Geometry check sheet. Reference: the model listing, model coordinates, mm. A direction names the side the tool comes from. Give positions to 0.01 mm unless a question says otherwise; leave off trailing zeros. Write each loop counter-clockwise with the first axis right and the second up, starting at its lowest first coordinate (ties: lowest second). Pieces come first, ordered by that corner, then holes. Notation, with made-up numbers: (71.5, 35) -> (119.5, 35) arc R20 cw to (119.5, 60) -> close; hole circle Ø11 at (60.25, -7). An arc over 180 degrees is marked (long way). One line per item, written item: value.
from build123d import *

# Parameters (mm, degrees)
CROQUIS1_R              = 2
SALIENTE_EXTRUIR1_DEPTH = 2.5
REDONDEO6_R             = 3
REDONDEO7_R             = 3
REDONDEO8_R             = 3


with BuildPart() as part:
    # Croquis1 → Saliente-Extruir1 (new body)
    with BuildSketch(Plane.XY):
        with BuildLine():
            Line((-15, 20.15), (-17.5, 20.15))
            Line((-17.5, 20.15), (-17.5, 15.15))
            Line((-17.5, 15.15), (-15, 15.15))
            Line((-15, 15.15), (-15, 10.15))
            Line((-15, 10.15), (-17.5, 10.15))
            Line((-17.5, 10.15), (-17.5, 0.15))
            Line((-17.5, 0.15), (-15, 0.15))
            Line((-15, 0.15), (-15, -9.85))
            Line((-15, -9.85), (-17.5, -9.85))
            Line((-17.5, -9.85), (-17.5, -19.85))
            Line((-17.5, -19.85), (-15, -19.85))
            Line((-15, -19.85), (-15, -24.85))
            Line((-15, -24.85), (-17.5, -24.85))
            Line((-17.5, -24.85), (-17.5, -29.85))
            Line((-17.5, -29.85), (-15, -29.85))
            Line((-15, -29.85), (15, -29.85))
            Line((15, -29.85), (17.5, -29.85))
            Line((17.5, -29.85), (17.5, -24.85))
            Line((17.5, -24.85), (15, -24.85))
            Line((15, -24.85), (15, -19.85))
            Line((15, -19.85), (17.5, -19.85))
            Line((17.5, -19.85), (17.5, -9.85))
            Line((17.5, -9.85), (15, -9.85))
            Line((15, -9.85), (15, 0.15))
            Line((15, 0.15), (17.5, 0.15))
            Line((17.5, 0.15), (17.5, 10.15))
            Line((17.5, 10.15), (15, 10.15))
            Line((15, 10.15), (15, 15.15))
            Line((15, 15.15), (17.5, 15.15))
            Line((17.5, 15.15), (17.5, 20.15))
            Line((17.5, 20.15), (15, 20.15))
            ThreePointArc((15, 20.15), (0, 35.15), (-15, 20.15))
        make_face()
        with Locations((-5, 24.315)):
            Circle(CROQUIS1_R, mode=Mode.SUBTRACT)
        with Locations((5, 24.315)):
            Circle(CROQUIS1_R, mode=Mode.SUBTRACT)
        with Locations((-5, -24.315)):
            Circle(CROQUIS1_R, mode=Mode.SUBTRACT)
        with Locations((5, -24.315)):
            Circle(CROQUIS1_R, mode=Mode.SUBTRACT)
        Polygon((-9.75, 20.15), (-1.5, 20.15), (-1.5, 26.15), (1.5, 26.15), (1.5, 20.15), (9.75, 20.15), (9.75, -20.15), (1.5, -20.15), (1.5, -26.15), (-1.5, -26.15), (-1.5, -20.15), (-9.75, -20.15), align=None, mode=Mode.SUBTRACT)
    extrude(amount=SALIENTE_EXTRUIR1_DEPTH)

    # Redondeo6
    redondeo6_edges = [part.edges().sort_by_distance(p)[0] for p in [
        (-1.5, -20.15, 1.25),
    ]]
    fillet(redondeo6_edges, radius=REDONDEO6_R)

    # Redondeo7
    redondeo7_edges = [part.edges().sort_by_distance(p)[0] for p in [
        (1.5, -20.15, 1.25),
    ]]
    fillet(redondeo7_edges, radius=REDONDEO7_R)

    # Redondeo8
    redondeo8_edges = [part.edges().sort_by_distance(p)[0] for p in [
        (1.5, 20.15, 1.25),
        (-1.5, 20.15, 1.25),
    ]]
    fillet(redondeo8_edges, radius=REDONDEO8_R)


solid = part.part
1) Sectioned sample at C-C on z = 0.4. Give the number of separate pieces and of enclosed holes in the cut face, plus the area to 3 significant figures.
Verdict:
separate pieces: 1
enclosed holes: 5
area: 1,120 mm^2
2) Tool access check on faces 1 (the flat face through (-16, 0.15, 1)), 2 (the flat face through (15, -5, 1)), 3 (the flat face through (-12, 3, 2.5)), 4 (the flat face through (0, -26.15, 1)). Record the directions out of +Z, -Z, +X, -X, +Y, -Y that give a thin tool (end or side, any length) a straight path to the whole face; none if there is none.
Verdict:
face 1: +Z, -Z, -X
face 2: +Z, -Z, +X
face 3: +Z, +X, -X, +Y, -Y
face 4: +Z, -Z
3) Sectioned sample at A-A on x = 0. Record the cut outline in (y, z), plus the area to 4 significant figures.
Verdict:
outline: (-29.85, 0) -> (-26.15, 0) -> (-26.15, 2.5) -> (-29.85, 2.5) -> close; (26.15, 0) -> (35.15, 0) -> (35.15, 2.5) -> (26.15, 2.5) -> close
area: 31.75 mm^2
4) Scan lines: probe 1 along Y at (x, z) = (15.5, 1); probe 2 along X at (y, z) = (-2.5, 0.25); probe 3 along X at (y, z) = (24.5, 1.9). Record each from-to range of solid material in increasing order.
Verdict:
probe 1: -29.85 to -24.85, -19.85 to -9.85, 0.15 to 10.15, 15.15 to 20.15
probe 2: -15 to -9.75, 9.75 to 15
probe 3: -14.36 to -6.99, -3.01 to -1.5, 1.5 to 3.01, 6.99 to 14.36
5) Depth check by flat-ended pin: pin 1 Ø12 at (x, y) = (9.5, 5.5) entering from -Z; pin 2 Ø0.8 at (x, z) = (-16, 1) entering from +Y; pin 3 Ø1.2 at (y, z) = (-3, 1) entering from +X; pin 4 Ø0.8 at (y, z) = (24.5, 1) entering from +X. Enter the tip coordinate at first touch or a pass-through.
Verdict:
pin 1: z = 0
pin 2: y = 20.15
pin 3: x = 15
pin 4: x = 14.47
6) Mould release check, pull along Y, two halves, no side actions. Record for faces 5 (the flat face through (-12, 3, 0)), 6 (the flat face through (9.75, 0, 1)), 7 (the flat face through (-1.5, -25, 1)): released by +Y, released by -Y, zero draft, split by the parting line, or undercut.
Verdict:
face 5: zero draft
face 6: undercut
face 7: undercut
7) Sectioned sample at B-B on y = 13. Record the cut outline in (x, z).
Verdict:
outline: (-15, 0) -> (-9.75, 0) -> (-9.75, 2.5) -> (-15, 2.5) -> close; (9.75, 0) -> (15, 0) -> (15, 2.5) -> (9.75, 2.5) -> close
